Source: CAD feature listing. Evaluate the final solid. Frame: model axes, mm. A direction names the side the tool comes from. Coordinates: 2 decimals unless noted, no trailing zeros. Order: outer loops, then holes, each group sorted by start corner. A loop starts at its lowest first (then second) coordinate and runs counter-clockwise, first axis right, second up.
```python
from build123d import *

# Parameters (mm, degrees)
SKETCH2_R               = 10.8712
BOSS_EXTRUDE2_DEPTH     = 30.1625
CUT_EXTRUDE1_DEPTH      = 11.176
CUT_EXTRUDE2_DEPTH      = 46.890822201
CIRPATTERN1_COUNT       = 2
FILLET1_R               = 5.55625
CUT_EXTRUDE3_DEPTH      = 46.890822336
CUT_EXTRUDE3_DEPTH_BACK = 46.890822336
SKETCH5_R               = 3.175
SKETCH7_W               = 23.3299
SKETCH7_H               = 14.3637
CUT_EXTRUDE5_DEPTH      = 23.7744
FILLET2_R               = 5.588


with BuildPart() as part:
    # Sketch2 → Boss-Extrude2 (new, symmetric)
    with BuildSketch(Plane(origin=(0, 0, 0), x_dir=(0, 0, -1), z_dir=(1, 0, 0))):
        with BuildLine():
            Line((-8.813470599, 9.906), (-10.99185, 9.906))
            Line((-10.99185, 9.906), (-13.716, 7.18185))
            Line((-13.716, 7.18185), (-13.716, 0))
            Line((-13.716, 0), (13.716, 0))
            Line((13.716, 0), (13.716, 7.18185))
            Line((13.716, 7.18185), (10.99185, 9.906))
            Line((10.99185, 9.906), (8.813470599, 9.906))
            ThreePointArc((8.813470599, 9.906), (0, 31.75), (-8.813470599, 9.906))
        make_face()
        with Locations(Location((0, 19.05, 0), (0, 0, 180))):
            Circle(SKETCH2_R, mode=Mode.SUBTRACT)
    extrude(amount=BOSS_EXTRUDE2_DEPTH, both=True)

    # Sketch3 → Cut-Extrude1 (cut, symmetric)
    with BuildSketch(Plane(origin=(0, 0, 0), x_dir=(0, 0, -1), z_dir=(1, 0, 0))):
        with BuildLine():
            Line((-8.813470599, 9.906), (-5.879647391, 9.906))
            ThreePointArc((-5.879647391, 9.906), (0, 29.9212), (5.879647391, 9.906))
            Line((5.879647391, 9.906), (8.813470599, 9.906))
            ThreePointArc((8.813470599, 9.906), (0, 31.75), (-8.813470599, 9.906))
        make_face()
    extrude(amount=CUT_EXTRUDE1_DEPTH, both=True, mode=Mode.SUBTRACT)

    # Sketch4 → Cut-Extrude2 (cut, through all)
    with BuildSketch(Plane(origin=(0, 0, 0), x_dir=(0, 0, -1), z_dir=(1, 0, 0))):
        with BuildLine():
            Line((-7.68709924, 26.73709924), (-8.980256121, 28.030256121))
            ThreePointArc((-8.980256121, 28.030256121), (-12.699462297, 18.933135262), (-8.813470599, 9.906))
            Line((-8.813470599, 9.906), (-5.879647391, 9.906))
            ThreePointArc((-5.879647391, 9.906), (-10.809053101, 17.889241411), (-7.68709924, 26.73709924))
        make_face()
    cut_extrude2 = extrude(amount=CUT_EXTRUDE2_DEPTH, mode=Mode.SUBTRACT)

    # CirPattern1: Cut-Extrude2 ×2 about axis
    cirpattern1_axis = Axis((0, 34.925, 0), (0, -1, 0))
    for i in range(1, CIRPATTERN1_COUNT):
        add(cut_extrude2.rotate(cirpattern1_axis, i * 360 / CIRPATTERN1_COUNT), mode=Mode.SUBTRACT)

    # Fillet1
    fillet1_edges = [part.edges().sort_by_distance(p)[0] for p in [
        (11.176, 27.38367768, 8.33367768),
        (30.1625, 27.38367768, 8.33367768),
        (-11.176, 27.38367768, -8.33367768),
        (-30.1625, 27.38367768, -8.33367768),
    ]]
    fillet(fillet1_edges, radius=FILLET1_R)

    # Mirror1: part across plane


with BuildPart() as part_1:
    add(part.part)
    add(part.part.mirror(Plane.ZX))

    # Sketch5 → Cut-Extrude3 (cut, two sides: drawn at the far end of the back side and taken through both)
    with BuildSketch(Plane(origin=(0, 0, 0), x_dir=(-1, 0, 0), z_dir=(0, 0, -1)).offset(-CUT_EXTRUDE3_DEPTH_BACK)):
        Circle(SKETCH5_R)
    extrude(amount=CUT_EXTRUDE3_DEPTH + CUT_EXTRUDE3_DEPTH_BACK, mode=Mode.SUBTRACT)

    # Cut-Extrude4 cone 1 section (through the dimple's axis) → Cut-Extrude4 (revolve, cut)
    with BuildSketch(Plane(origin=(0, 0, -13.716), x_dir=(0, 1, 0), z_dir=(1, 0, 0))):
        Polygon((0, 0), (6.223, 0), (0, 6.223), align=None)
    revolve(axis=Axis((0, 0, -13.716), (0, 0, 1)), mode=Mode.SUBTRACT)

    # Sketch7 → Cut-Extrude5 (cut)
    with BuildSketch(Plane.XY.offset(13.716)):
        with Locations((-16.66875, 0)):
            Rectangle(SKETCH7_W, SKETCH7_H)
        with Locations((16.66875, 0)):
            Rectangle(SKETCH7_W, SKETCH7_H)
    extrude(amount=-CUT_EXTRUDE5_DEPTH, mode=Mode.SUBTRACT)

    # Fillet2
    fillet2_edges = [part_1.edges().sort_by_distance(p)[0] for p in [
        (11.176, -9.906, -7.346558995),
        (-11.176, -9.906, 7.346558995),
        (-11.176, 9.906, 7.346558995),
        (11.176, 9.906, -7.346558995),
    ]]
    fillet(fillet2_edges, radius=FILLET2_R)


solid = part_1.part
```
Q1. Section query B-B on z = 0. Give the number of separate pieces and of enclosed holes in the cut face, plus the area to 3 significant figures.
Solutions:
separate pieces: 5
enclosed holes: 3
area: 424 mm2
Q2. Material intervals for line 1 along Y through (x, z) = (-15.5, 0); line 2 along X through (y, z) = (0, 1) (1 decimal); line 3 along Y through (x, z) = (-13.5, -9.75), sorted ascending.
Solutions:
line 1: y = -31.75 to -29.92, -8.18 to -7.18, 7.18 to 8.18, 29.92 to 31.75
line 2: x = -30.2 to -28.3, -5 to -3.2, 3.2 to 5, 28.3 to 30.2
line 3: y = -9.91 to -7.18, 7.18 to 9.91
Q3. Section query A-A on y = 0. Output: boundary loops of the cut face in (x, z) (1 decimal), plus the area to 3 significant figures.
Solutions:
outline: (-30.2, -13.7) - (-6.2, -13.7) - (-3.2, -10.7) - (-3.2, 13.7) - (-5, 13.7) - (-5, -10.1) - (-28.3, -10.1) - (-28.3, 13.7) - (-30.2, 13.7) - close; (3.2, -10.7) - (6.2, -13.7) - (30.2, -13.7) - (30.2, 13.7) - (28.3, 13.7) - (28.3, -10.1) - (5, -10.1) - (5, 13.7) - (3.2, 13.7) - close
area: 362 mm2
Q4. Pull-direction query (Y, two-part tool) for faces 1 (the cylindrical face through (-12.76, -28.305, -6.893)), 2 (the cylindrical face through (-9.583, -11.586, 8.992)), 3 (the cylindrical face through (9.496, 11.499, -9.08)); classes: pulls with the +Y half, pulls with the -Y half, needs draft (parallel to the pull), parting line crosses it, or undercut.
Solutions:
face 1: undercut
face 2: pulls with the -Y half
face 3: pulls with the +Y half
Q5. Section query C-C on x = 0. Output: boundary loops of the cut face in (y, z) (3 decimals), plus the area to 3 significant figures.
Solutions:
outline: (-9.906, -10.992) - (-7.182, -13.716) - (-6.223, -13.716) - (-3.175, -10.668) - (-3.175, 13.716) - (-7.182, 13.716) - (-9.906, 10.992) - (-9.906, 5.88) arc R10.871 cw to (-9.906, -5.88) - close; (3.175, -10.668) - (6.223, -13.716) - (7.182, -13.716) - (9.906, -10.992) - (9.906, -5.88) arc R10.871 cw to (9.906, 5.88) - (9.906, 10.992) - (7.182, 13.716) - (3.175, 13.716) - close
area: 318 mm2
Q6. Pin query (flat end, axial travel): P1, Ø10, axis at x = -5.5, z = 6.5, coming from the -Y side; P2, Ø13, axis at y = 19.05, z = 0, coming from the -X side; P3, Ø1.5, axis at x = -23, z = -2, coming from the -Y side; P4, Ø4, axis at x = -4.5, z = -3, coming from the +Y side. Return the tip coordinate at first contact, or that it passes through.
Solutions:
P1: stops at y = -12.21
P2: passes through
P3: stops at y = -31.69
P4: stops at y = 9.4
Q7. Section query D-D on y = 23. Output: boundary loops of the cut face in (x, z), plus the area to 3 significant figures.
Solutions:
outline: (-30.16, 10.13) - (-11.18, 10.13) - (-11.18, 12.07) - (-30.16, 12.07) - close; (11.18, -12.07) - (30.16, -12.07) - (30.16, -10.13) - (11.18, -10.13) - close
area: 73.7 mm2
Q8. Set-up query: faces 4 (the cylindrical face through (-12.76, 28.305, -6.893)), 5 (the flat face through (17, 7.182, 2)), 6 (the cylindrical face through (28.5, -28.2, 6.9)). Return all of +Z, -Z, +X, -X, +Y, -Y with unobstructed straight access to the full face (end or side cutting, diameter ignored); none if empty.
Solutions:
face 4: -Z
face 5: +Z
face 6: +Z, +X
